Model file for the job. Use its own axes, mm. Face numbers are marked on the shaded views. A direction names the side the tool comes from. Round coordinates to 2 decimals unless told otherwise and drop trailing zeros. Put each result on its own line as item: value. Start each with the question number.
Item 1: Pin check, flat tips, straight feed: pin 1 Ø0.8 at (x, z) = (1, 6) entering from +Y; pin 2 Ø10 at (x, y) = (-2.5, 13) entering from +Z; pin 3 Ø3 at (y, z) = (28, -2.5) entering from -X. Stop position of each tip, or through.
Item 2: Mould opens along Z. For the marked faces 1, 2 and 3 say: pulls with the +Z half, pulls with the -Z half, needs draft (parallel to the pull), parting line crosses it, or undercut.
Item 3: Probe probe 1 along Y at (x, z) = (2.25, 6.75); probe 2 along Y at (x, z) = (-7.25, -6.75); probe 3 along Y at (x, z) = (8.5, 6). List the from-to ranges inside material, lowest first.
Item 4: Saw through at A-A on y = 38.1. State how many separate pieces and enclosed holes the cut face has, plus the area to 3 significant figures.
Item 5: Which spindle directions (+Z, -Z, +X, -X, +Y, -Y) get a long thin tool onto all of the face, cutting with end or side? Do the marked faces 4, 5 and 6. Say none if no direction does.
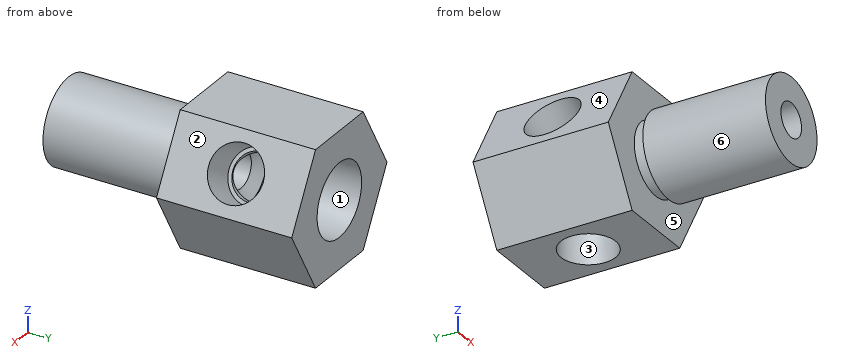
```python
from build123d import *
from OCP.BRepAlgoAPI import BRepAlgoAPI_Cut
from OCP.TopTools import TopTools_ListOfShape

# Parameters (mm, degrees)
SKETCH1_R           = 7.9375
BOSS_EXTRUDE1_DEPTH = 25.4
BOSS_EXTRUDE2_DEPTH = 25.4
SKETCH3_R           = 3.175
CUT_EXTRUDE1_DEPTH  = 55.37815125
SKETCH6_R           = 6.6675
CUT_EXTRUDE2_DEPTH  = 2.38125


with BuildPart() as part:
    # Sketch1 → Boss-Extrude1 (new body)
    with BuildSketch(Plane(origin=(0, 0, 0), x_dir=(1, 0, 0), z_dir=(0, 1, 0))):
        with Locations(Location((0, 0, 0), (0, 0, 270))):
            Circle(SKETCH1_R)
    extrude(amount=BOSS_EXTRUDE1_DEPTH)

    # Sketch2 → Boss-Extrude2 (add)
    with BuildSketch(Plane(origin=(0, 25.4, 0), x_dir=(1, 0, 0), z_dir=(0, 1, 0))):
        Polygon((14.664696837, 0), (7.332348419, 12.7), (-7.332348419, 12.7), (-14.664696837, 0), (-7.332348419, -12.7), (7.332348419, -12.7), align=None)
    extrude(amount=BOSS_EXTRUDE2_DEPTH)

    # Sketch3 → Cut-Extrude1 (cut, through all)
    with BuildSketch(Plane.XZ):
        with Locations(Location((0, 0, 0), (0, 0, 270))):
            Circle(SKETCH3_R)
    extrude(amount=-CUT_EXTRUDE1_DEPTH, mode=Mode.SUBTRACT)

    # Sketch6 → Cut-Extrude2 (cut)
    with BuildSketch(Plane.XZ.offset(-25.4)):
        Polygon((-14.664696837, 0), (-7.332348419, 12.7), (7.332348419, 12.7), (14.664696837, 0), (7.332348419, -12.7), (-7.332348419, -12.7), align=None)
        with Locations(Location((0, 0, 0), (0, 0, 90))):
            Circle(SKETCH6_R, mode=Mode.SUBTRACT)
    extrude(amount=CUT_EXTRUDE2_DEPTH, mode=Mode.SUBTRACT)

    # Sketch4 → 1_4 NPT Tapped Hole1 (revolve, cut)
    with BuildSketch(Plane(origin=(0, 50.8, 0), x_dir=(0, 0, 1), z_dir=(1, 0, 0))):
        Polygon((0, 0), (0, 20.360347279), (5.5626, 17.018), (5.5626, 9.906), (6.557984794, 9.906), (6.8545837, 0), align=None)
    revolve(axis=Axis((0, 57.15, 0), (0, -1, 0)), mode=Mode.SUBTRACT)


with BuildPart() as f_1_8_npt_tapped_hole1_tool:
    # Sketch9 → 1_8 NPT Tapped Hole1 (revolve)
    with BuildSketch(Plane(origin=(10.998522628, 38.1, 6.35), x_dir=(0.4999999999999991, 0, -0.8660254037844392), z_dir=(0, 1, 0))):
        Polygon((0, 0), (0, 14.217468714), (4.2164, 11.684), (4.2164, 6.858), (4.936181096, 6.858), (5.1415188, 0), align=None)
    revolve(axis=Axis((16.497783942, 38.1, 9.525), (-0.8660254037844392, 0, -0.4999999999999991)))


with BuildPart() as part_1:
    add(part.part)

    # 1_8 NPT Tapped Hole1: cut by f_1_8_npt_tapped_hole1_tool, with a tolerance
    f_1_8_npt_tapped_hole1_stock = TopTools_ListOfShape()
    f_1_8_npt_tapped_hole1_stock.Append(part_1.part.wrapped)
    f_1_8_npt_tapped_hole1_tools = TopTools_ListOfShape()
    f_1_8_npt_tapped_hole1_tools.Append(f_1_8_npt_tapped_hole1_tool.part.wrapped)
    f_1_8_npt_tapped_hole1_cut = BRepAlgoAPI_Cut()
    f_1_8_npt_tapped_hole1_cut.SetArguments(f_1_8_npt_tapped_hole1_stock)
    f_1_8_npt_tapped_hole1_cut.SetTools(f_1_8_npt_tapped_hole1_tools)
    f_1_8_npt_tapped_hole1_cut.SetFuzzyValue(0.00001)
    f_1_8_npt_tapped_hole1_cut.Build()
    add(Compound.cast(f_1_8_npt_tapped_hole1_cut.Shape()).solids(), mode=Mode.REPLACE)


with BuildPart() as f_1_8_npt_tapped_hole1_at_2_tool:
    # Sketch9 at point 2 (on carried to point 2, square into its face) → 1_8 NPT Tapped Hole1 at 2 (revolve)
    with BuildSketch(Plane(origin=(0, 38.1, -12.7), x_dir=(-1, 0, 0), z_dir=(0, 1, 0))):
        Polygon((0, 0), (0, 14.217468714), (4.2164, 11.684), (4.2164, 6.858), (4.936181096, 6.858), (5.1415188, 0), align=None)
    revolve(axis=Axis((0, 38.1, -19.05), (0, 0, 1)))


with BuildPart() as part_2:
    add(part_1.part)

    # 1_8 NPT Tapped Hole1 at 2: cut by f_1_8_npt_tapped_hole1_at_2_tool, with a tolerance
    f_1_8_npt_tapped_hole1_at_2_stock = TopTools_ListOfShape()
    f_1_8_npt_tapped_hole1_at_2_stock.Append(part_2.part.wrapped)
    f_1_8_npt_tapped_hole1_at_2_tools = TopTools_ListOfShape()
    f_1_8_npt_tapped_hole1_at_2_tools.Append(f_1_8_npt_tapped_hole1_at_2_tool.part.wrapped)
    f_1_8_npt_tapped_hole1_at_2_cut = BRepAlgoAPI_Cut()
    f_1_8_npt_tapped_hole1_at_2_cut.SetArguments(f_1_8_npt_tapped_hole1_at_2_stock)
    f_1_8_npt_tapped_hole1_at_2_cut.SetTools(f_1_8_npt_tapped_hole1_at_2_tools)
    f_1_8_npt_tapped_hole1_at_2_cut.SetFuzzyValue(0.00001)
    f_1_8_npt_tapped_hole1_at_2_cut.Build()
    add(Compound.cast(f_1_8_npt_tapped_hole1_at_2_cut.Shape()).solids(), mode=Mode.REPLACE)


with BuildPart() as f_1_8_npt_tapped_hole1_at_3_tool:
    # Sketch9 at point 3 (on carried to point 3, square into its face) → 1_8 NPT Tapped Hole1 at 3 (revolve)
    with BuildSketch(Plane(origin=(-10.998522628, 38.1, 6.35), x_dir=(0.500000175, 0, 0.866025303), z_dir=(0, 1, 0))):
        Polygon((0, 0), (0, 14.217468714), (4.2164, 11.684), (4.2164, 6.858), (4.936181096, 6.858), (5.1415188, 0), align=None)
    revolve(axis=Axis((-16.497783301, 38.1, 9.52500111), (0.866025303, 0, -0.500000175)))


with BuildPart() as part_3:
    add(part_2.part)

    # 1_8 NPT Tapped Hole1 at 3: cut by f_1_8_npt_tapped_hole1_at_3_tool, with a tolerance
    f_1_8_npt_tapped_hole1_at_3_stock = TopTools_ListOfShape()
    f_1_8_npt_tapped_hole1_at_3_stock.Append(part_3.part.wrapped)
    f_1_8_npt_tapped_hole1_at_3_tools = TopTools_ListOfShape()
    f_1_8_npt_tapped_hole1_at_3_tools.Append(f_1_8_npt_tapped_hole1_at_3_tool.part.wrapped)
    f_1_8_npt_tapped_hole1_at_3_cut = BRepAlgoAPI_Cut()
    f_1_8_npt_tapped_hole1_at_3_cut.SetArguments(f_1_8_npt_tapped_hole1_at_3_stock)
    f_1_8_npt_tapped_hole1_at_3_cut.SetTools(f_1_8_npt_tapped_hole1_at_3_tools)
    f_1_8_npt_tapped_hole1_at_3_cut.SetFuzzyValue(0.00001)
    f_1_8_npt_tapped_hole1_at_3_cut.Build()
    add(Compound.cast(f_1_8_npt_tapped_hole1_at_3_cut.Shape()).solids(), mode=Mode.REPLACE)


solid = part_3.part
```
Results found:
1. pin 1: stops at y = 40.89
1. pin 2: stops at z = 7.94
1. pin 3: stops at x = -14.09
2. face 1: undercut
2. face 2: pulls with the +Z half
2. face 3: pulls with the -Z half
3. probe 1: y = 0 to 23.02, 25.4 to 50.8
3. probe 2: y = 25.4 to 50.8
3. probe 3: y = 25.4 to 33.12, 43.08 to 50.8
4. separate pieces: 3
4. enclosed holes: 0
4. area: 232 mm²
5. face 4: +Z, -X, +Y, -Y
5. face 5: none
5. face 6: -Y
